Source: three-view drawing plus pictorial views. Frame: mm from the lowest corner of the part. A direction names the side the tool comes from. Give positions to 0.01 mm unless a question says otherwise; leave off trailing zeros. Order: outer loops, then holes, each group sorted by start corner. A loop starts at its lowest first (then second) coordinate and runs counter-clockwise, first axis right, second up. Notation, with made-up numbers: (-34.5, -26.5) - (9.5, -26.5) arc R25 ccw to (9.5, -6.5) - close; hole circle Ø11 at (14, 6.5). An arc over 180 degrees is marked (long way). Answer in a Markdown table with one row per item. Add a question column.
1. Mould query, pull axis X, two halves, no side actions, for the marked faces 4, 5, 6 and 7. Classes: released by +X, released by -X, zero draft, split by the parting line, or undercut.
2. Ray query, line 1 (Z direction, x = 6.5, y = 9.75); line 2 (X direction, y = 3, z = 2.75); line 3 (Z direction, x = 0.75, y = 7). Return the intervals inside material, ascending. Write a range as [from, to].
3. Section query B-B on y = 7. Return loops of the section in (x, z).
4. Section query C-C on z = 1.6. Return loops of the section in (x, y), and give its area (3 significant figures).
5. Section query A-A on x = 3.5. Return loops of the section in (y, z), and give its area (3 significant figures).
6. Access query for the marked faces 1, 2 and 3. Directions: +Z, -Z, +X, -X, +Y, -Y. A direction counts if a zero-diameter tool reaches every point of the face in a straight line with its end or side. Return the directions, or none.
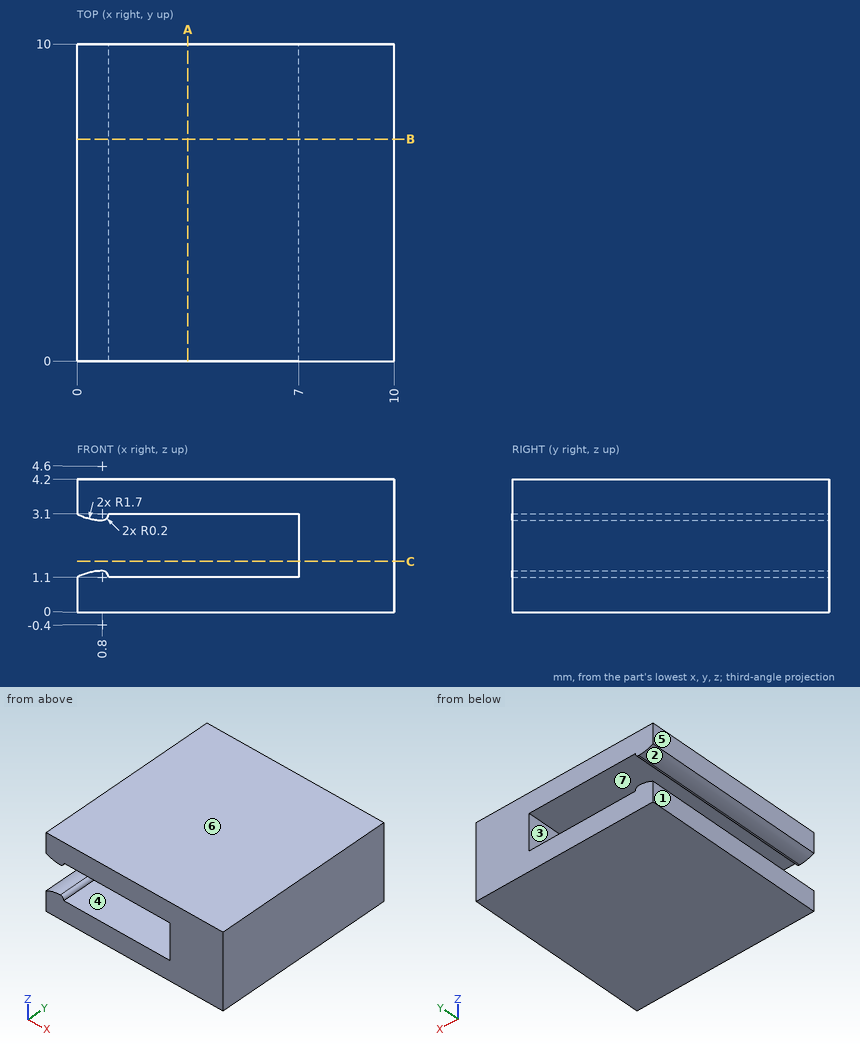
Answer:
| question | item | result |
|---|---|---|
| 1 | face 4 | undercut |
| 1 | face 5 | released by -X |
| 1 | face 6 | zero draft |
| 1 | face 7 | undercut |
| 2 | line 1 | z = [0, 1.1], [3.1, 4.2] |
| 2 | line 2 | x = [7, 10] |
| 2 | line 3 | z = [0, 1.3], [2.9, 4.2] |
| 3 | outline | (0, 0) - (10, 0) - (10, 4.2) - (0, 4.2) - (0, 3.1) arc R1.7 ccw to (0.8, 2.9) arc R0.2 ccw to (1, 3.1) - (7, 3.1) - (7, 1.1) - (1, 1.1) arc R0.2 ccw to (0.8, 1.3) arc R1.7 ccw to (0, 1.1) - close |
| 4 | outline | (7, 0) - (10, 0) - (10, 10) - (7, 10) - close |
| 4 | area | 30.0 mm² |
| 5 | outline | (0, 0) - (10, 0) - (10, 1.1) - (0, 1.1) - close; (0, 3.1) - (10, 3.1) - (10, 4.2) - (0, 4.2) - close |
| 5 | area | 22.0 mm² |
| 6 | face 1 | +Z, -Z, -X, +Y, -Y |
| 6 | face 2 | -X, +Y, -Y |
| 6 | face 3 | +Y, -Y |
